Geometry check sheet. Reference: the model listing, model coordinates, mm. Face numbers are marked on the shaded views. A direction names the side the tool comes from. Give positions to 0.01 mm unless a question says otherwise; leave off trailing zeros. Loops run counter-clockwise (first coordinate to the right, second up) from the corner with the lowest first, then second, coordinate; pieces in that order, holes last. Notation, with made-up numbers: (3, 82) -> (25, 82) arc R14 ccw to (25, 104) -> close; hole circle Ø6 at (17.25, 54). An arc over 180 degrees is marked (long way). Write each question's results on one line, items separated by ' | '. Start each with the question number.
1) Scan lines: line 1 (Z direction, x = -21, y = -25); line 2 (Z direction, x = -19, y = -148); line 3 (X direction, y = -153.5, z = -38). Record each from-to range of solid material in increasing order. Write a range as from..to.
2) Set-up check for the marked faces 1, 2 and 3: record each of +Z, -Z, +X, -X, +Y, -Y from which the full face is reachable in a straight line by a thin tool's end or side.
3) Draft check along X on the marked faces 4, 5 and 6. Enter one of: pulls with the +X half, pulls with the -X half, needs draft (parallel to the pull), parting line crosses it, or undercut.
4) Sectioned sample at B-B on x = -11. Record the cut outline in (y, z).
5) Sectioned sample at D-D on z = -38.5. Record the cut outline in (x, y), then the cut area to 3 significant figures.
6) Sectioned sample at C-C on z = -3.5. Record the cut outline in (x, y).
7) Depth check by flat-ended pin: pin 1 (1.4 mm diameter, centred on y = -144.5, z = -17, fed in from +X); pin 2 (1 mm diameter, centred on x = -5.5, z = -44, fed in from +Y); pin 3 (8 mm diameter, centred on y = -164, z = -5, fed in from -X). Enter the tip coordinate at first touch or a pass-through.
8) Sectioned sample at A-A on y = -148. Record the cut outline in (x, z).
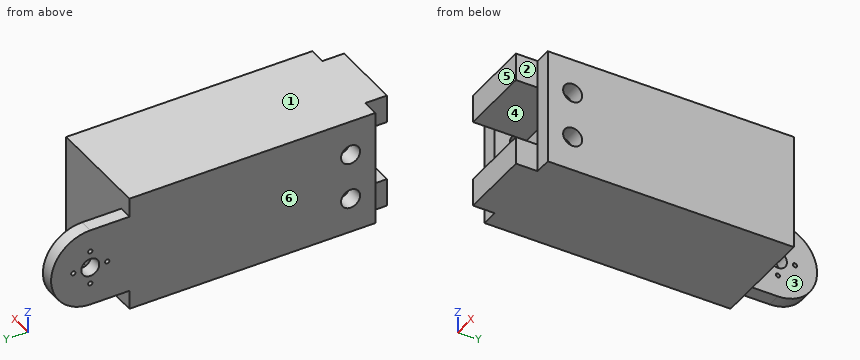
```python
from build123d import *

# Parameters (mm, degrees)
SKETCH1_W               = 50
SKETCH1_H               = 150
BOSS_EXTRUDE1_DEPTH     = 55
CUT_EXTRUDE1_DEPTH      = 168.406690428
CUT_EXTRUDE1_DEPTH_BACK = 45
SKETCH2_R               = 10.25
SKETCH7_R               = 1
SKETCH7_R_2             = 4.25
CUT_EXTRUDE3_DEPTH      = 10
SKETCH8_W               = 55
SKETCH8_H               = 55
SKETCH8_R               = 10.25
BOSS_EXTRUDE2_DEPTH     = 50
SKETCH10_W              = 8
SKETCH10_H              = 10.25
SKETCH10_W_2            = 17
SKETCH10_H_2            = 1
SKETCH10_W_3            = 34
SKETCH10_H_3            = 20
SKETCH10_H_4            = 5
CUT_EXTRUDE4_DEPTH      = 214.717102732
SKETCH11_W              = 34
SKETCH11_H              = 13.25
BOSS_EXTRUDE4_DEPTH     = 25
SKETCH13_W              = 55
SKETCH13_H              = 10
CUT_EXTRUDE5_DEPTH      = 8
SKETCH14_R              = 5.030159043
CUT_EXTRUDE6_DEPTH      = 8
SKETCH15_W              = 34
SKETCH15_H              = 0.25
BOSS_EXTRUDE5_DEPTH     = 13.25
CUT_EXTRUDE7_DEPTH      = 181.416185527
BOSS_EXTRUDE6_START     = 1.5
SKETCH19_R              = 10.25
SKETCH19_R_2            = 1
SKETCH19_R_3            = 4.25
BOSS_EXTRUDE6_DEPTH     = 1.5
CUT_EXTRUDE8_DEPTH      = 184.89467094
SKETCH21_R              = 5.030159043
SKETCH21_R_2            = 4.5
BOSS_EXTRUDE7_DEPTH     = 8


with BuildPart() as part:
    # Sketch1 → Boss-Extrude1 (new body)
    with BuildSketch(Plane.XY):
        with Locations((0, -75)):
            Rectangle(SKETCH1_W, SKETCH1_H)
    extrude(amount=-BOSS_EXTRUDE1_DEPTH)

    # Sketch2 → Cut-Extrude1 (cut, two sides: drawn at the far end of the back side and taken through both)
    with BuildSketch(Plane(origin=(25, 0, 0), x_dir=(0, 0, -1), z_dir=(1, 0, 0)).offset(-CUT_EXTRUDE1_DEPTH_BACK)):
        with Locations(Location((27.5, -25, 0), (0, 0, 270))):
            Circle(SKETCH2_R)
    extrude(amount=CUT_EXTRUDE1_DEPTH + CUT_EXTRUDE1_DEPTH_BACK, mode=Mode.SUBTRACT)

    # Sketch7 → Cut-Extrude3 (cut)
    with BuildSketch(Plane(origin=(-20, 0, 0), x_dir=(0, 0, -1), z_dir=(1, 0, 0))):
        with Locations(Location((27.5, -17, 0), (0, 0, 90))):
            Circle(SKETCH7_R)
        with Locations(Location((35.5, -25, 0), (0, 0, 90))):
            Circle(SKETCH7_R)
        with Locations(Location((27.5, -33, 0), (0, 0, 90))):
            Circle(SKETCH7_R)
        with Locations(Location((19.5, -25, 0), (0, 0, 90))):
            Circle(SKETCH7_R)
        with Locations(Location((27.5, -25, 0), (0, 0, 90))):
            Circle(SKETCH7_R_2)
    extrude(amount=-CUT_EXTRUDE3_DEPTH, mode=Mode.SUBTRACT)

    # Sketch8 → Boss-Extrude2 (add)
    with BuildSketch(Plane(origin=(25, 0, 0), x_dir=(0, 0, -1), z_dir=(1, 0, 0))):
        with Locations((27.5, -177.5)):
            Rectangle(SKETCH8_W, SKETCH8_H)
        with Locations(Location((27.5, -180, 0), (0, 0, 90))):
            Circle(SKETCH8_R, mode=Mode.SUBTRACT)
    extrude(amount=-BOSS_EXTRUDE2_DEPTH)

    # Sketch10 → Cut-Extrude4 (cut, through all)
    with BuildSketch(Plane.XY):
        Polygon((-17, -205), (17, -205), (17, -191.25), (0, -191.25), (-17, -191.25), align=None)
        Polygon((-25, -205), (-17, -205), (-17, -191.25), (-17, -190.25), (-25, -190.25), align=None)
        Polygon((17, -191.25), (17, -205), (25, -205), (25, -190.25), (17, -190.25), align=None)
        with Locations((-21, -185.125)):
            Rectangle(SKETCH10_W, SKETCH10_H)
        with Locations((-21, -174.875)):
            Rectangle(SKETCH10_W, SKETCH10_H)
        with Locations((21, -174.875)):
            Rectangle(SKETCH10_W, SKETCH10_H)
        with Locations((21, -185.125)):
            Rectangle(SKETCH10_W, SKETCH10_H)
        with Locations((-8.5, -185.125)):
            Rectangle(SKETCH10_W_2, SKETCH10_H)
        with Locations((8.5, -185.125)):
            Rectangle(SKETCH10_W_2, SKETCH10_H)
        Polygon((0, -180), (17, -180), (17, -169.75), (-17, -169.75), (-17, -180), align=None)
        with Locations((-8.5, -190.75)):
            Rectangle(SKETCH10_W_2, SKETCH10_H_2)
        with Locations((8.5, -190.75)):
            Rectangle(SKETCH10_W_2, SKETCH10_H_2)
        with Locations((0, -154.75)):
            Rectangle(SKETCH10_W_3, SKETCH10_H_3)
        with Locations((0, -167.25)):
            Rectangle(SKETCH10_W_3, SKETCH10_H_4)
    extrude(amount=-CUT_EXTRUDE4_DEPTH, mode=Mode.SUBTRACT)

    # Sketch11 → Boss-Extrude4 (add)
    with BuildSketch(Plane.XZ.offset(144.75)):
        with Locations((0, -6.625)):
            Rectangle(SKETCH11_W, SKETCH11_H)
        with Locations((0, -48.375)):
            Rectangle(SKETCH11_W, SKETCH11_H)
    extrude(amount=BOSS_EXTRUDE4_DEPTH)

    # Sketch13 → Cut-Extrude5 (cut)
    with BuildSketch(Plane(origin=(25, 0, 0), x_dir=(0, 0, -1), z_dir=(1, 0, 0))):
        with Locations((27.5, -164.75)):
            Rectangle(SKETCH13_W, SKETCH13_H)
    cut_extrude5 = extrude(amount=-CUT_EXTRUDE5_DEPTH, mode=Mode.SUBTRACT)

    # Mirror2: Cut-Extrude5 across plane
    add(cut_extrude5.mirror(Plane(origin=(0, 0, 0), x_dir=(0, 0, 1), z_dir=(1, 0, 0))), mode=Mode.SUBTRACT)

    # Sketch14 → Cut-Extrude6 (cut)
    with BuildSketch(Plane(origin=(25, 0, 0), x_dir=(0, 0, -1), z_dir=(1, 0, 0))):
        with Locations(Location((16.5, -148, 0), (0, 0, 90))):
            Circle(SKETCH14_R)
        with Locations(Location((38.5, -148, 0), (0, 0, 90))):
            Circle(SKETCH14_R)
    cut_extrude6 = extrude(amount=-CUT_EXTRUDE6_DEPTH, mode=Mode.SUBTRACT)

    # Mirror3: Cut-Extrude6 across plane
    add(cut_extrude6.mirror(Plane(origin=(0, 0, 0), x_dir=(0, 0, 1), z_dir=(1, 0, 0))), mode=Mode.SUBTRACT)

    # Sketch15 → Boss-Extrude5 (add)
    with BuildSketch(Plane.XY):
        with Locations((0, -169.875)):
            Rectangle(SKETCH15_W, SKETCH15_H)
    boss_extrude5 = extrude(amount=-BOSS_EXTRUDE5_DEPTH)

    # Mirror4: Boss-Extrude5 across plane
    add(boss_extrude5.mirror(Plane.XY.offset(-27.5)))

    # Sketch16 → Cut-Extrude7 (cut, through all)
    with BuildSketch(Plane.XY):
        Polygon((-18.5, 0), (-18.5, -14.75), (-18.5, -35.25), (-18.5, -43.5), (25, -43.5), (25, 0), align=None)
    extrude(amount=-CUT_EXTRUDE7_DEPTH, mode=Mode.SUBTRACT)

    # Sketch19 → Boss-Extrude6 (add)
    with BuildSketch(Plane(origin=(-20, 0, 0), x_dir=(0, 0, -1), z_dir=(1, 0, 0)).offset(BOSS_EXTRUDE6_START)):
        with Locations((27.5, -25)):
            Circle(SKETCH19_R)
        with Locations(Location((27.5, -17, 0), (0, 0, 90))):
            Circle(SKETCH19_R_2, mode=Mode.SUBTRACT)
        with Locations(Location((27.5, -33, 0), (0, 0, 90))):
            Circle(SKETCH19_R_2, mode=Mode.SUBTRACT)
        with Locations(Location((19.5, -25, 0), (0, 0, 90))):
            Circle(SKETCH19_R_2, mode=Mode.SUBTRACT)
        with Locations(Location((35.5, -25, 0), (0, 0, 90))):
            Circle(SKETCH19_R_2, mode=Mode.SUBTRACT)
        with Locations(Location((27.5, -25, 0), (0, 0, 90))):
            Circle(SKETCH19_R_3, mode=Mode.SUBTRACT)
    extrude(amount=-BOSS_EXTRUDE6_DEPTH)

    # Sketch20 → Cut-Extrude8 (cut, through all)
    with BuildSketch(Plane(origin=(-18.5, 0, 0), x_dir=(0, 0, -1), z_dir=(1, 0, 0))):
        with BuildLine():
            Line((0, 0), (0, -43.5))
            Line((0, -43.5), (9, -43.5))
            Line((9, -43.5), (9, -25))
            ThreePointArc((9, -25), (27.5, -6.5), (46, -25))
            Line((46, -25), (46, -43.5))
            Line((46, -43.5), (55, -43.5))
            Line((55, -43.5), (55, 0))
            Line((55, 0), (0, 0))
        make_face()
    extrude(amount=-CUT_EXTRUDE8_DEPTH, mode=Mode.SUBTRACT)

    # Sketch21 → Boss-Extrude7 (add)
    # profile 1 of 2: a face of its own
    with BuildSketch(Plane(origin=(25, 0, 0), x_dir=(0, 0, -1), z_dir=(1, 0, 0))):
        with Locations(Location((16.5, -148, 0), (0, 0, 229.751587581))):
            Circle(SKETCH21_R)
        with Locations(Location((16.5, -148, 0), (0, 0, 90))):
            Circle(SKETCH21_R_2, mode=Mode.SUBTRACT)
    # profile 2 of 2: a face of its own
    with BuildSketch(Plane(origin=(25, 0, 0), x_dir=(0, 0, -1), z_dir=(1, 0, 0))):
        with Locations(Location((38.5, -148, 0), (0, 0, 310.248412419))):
            Circle(SKETCH21_R)
        with Locations(Location((38.5, -148, 0), (0, 0, 90))):
            Circle(SKETCH21_R_2, mode=Mode.SUBTRACT)
    boss_extrude7 = extrude(amount=-BOSS_EXTRUDE7_DEPTH)

    # Mirror5: Boss-Extrude7 across plane
    add(boss_extrude7.mirror(Plane(origin=(0, 0, 0), x_dir=(0, 0, 1), z_dir=(1, 0, 0))))


solid = part.part
```
Result:
1) line 1: -46..-36.5, -34.5..-31.75, -23.25..-20.5, -18.5..-9 | line 2: -55..-43, -34..-21, -12..0 | line 3: -25..-17, 17..25
2) face 1: +Z, +X, -X, +Y, -Y | face 2: +Z, -Z, +X, -Y | face 3: +Z, -Z, +X, +Y
3) face 4: undercut | face 5: needs draft | face 6: pulls with the -X half
4) outline: (-170, -55) -> (-43.5, -55) -> (-43.5, 0) -> (-170, 0) -> (-170, -13.25) -> (-144.75, -13.25) -> (-144.75, -41.75) -> (-170, -41.75) -> close
5) outline: (-25, -159.75) -> (-17, -159.75) -> (-17, -152.5) -> (-25, -152.5) -> close; (-25, -143.5) -> (-17, -143.5) -> (-17, -144.75) -> (17, -144.75) -> (17, -143.5) -> (25, -143.5) -> (25, -43.5) -> (-18.5, -43.5) -> (-18.5, -10.13) -> (-25, -10.13) -> close; (17, -159.75) -> (25, -159.75) -> (25, -152.5) -> (17, -152.5) -> close | area: 5,380 mm^2
6) outline: (-25, -159.75) -> (-17, -159.75) -> (-17, -170) -> (17, -170) -> (17, -159.75) -> (25, -159.75) -> (25, -43.5) -> (-25, -43.5) -> close
7) pin 1: x = 17 | pin 2: y = -43.5 | pin 3: x = -17
8) outline: (-25, -55) -> (25, -55) -> (25, -43) -> (17, -43) -> (17, -41.75) -> (-17, -41.75) -> (-17, -43) -> (-25, -43) -> close; (-25, -34) -> (-17, -34) -> (-17, -21) -> (-25, -21) -> close; (-25, -12) -> (-17, -12) -> (-17, -13.25) -> (17, -13.25) -> (17, -12) -> (25, -12) -> (25, 0) -> (-25, 0) -> close; (17, -34) -> (25, -34) -> (25, -21) -> (17, -21) -> close
